The listing builds one solid part. Answer for the finished solid, in the listing's coordinates (mm). A direction names the side the tool comes from. Round coordinates to 2 decimals unless told otherwise and drop trailing zeros. Loops run counter-clockwise (first coordinate to the right, second up) from the corner with the lowest first, then second, coordinate; pieces in that order, holes last. Notation, with made-up numbers: (4, -5) -> (56, -5) arc R27 cw to (56, 30) -> close; hole circle Ø2 at (-11, 17.5). An arc over 180 degrees is marked (long way). One line per question, with ' | ' between items.
from build123d import *

# Parameters (mm, degrees)
BOX_W                   = 3.1
BOX_H                   = 13
BOX_DEPTH               = 12
BOX001_W                = 3.1
BOX001_H                = 10
BOX001_DEPTH            = 5
BOX002_W                = 3.1
BOX002_H                = 10
BOX002_DEPTH            = 5
CYLINDER_R              = 2.75
CYLINDER_DEPTH          = 3.1
CYLINDER_PITCH_ANGLE    = 90
CYLINDER001_R           = 2.75
CYLINDER001_DEPTH       = 3.06
CYLINDER001_PITCH_ANGLE = 90
PAD001_DEPTH            = 41
POCKET_DEPTH            = 41


with BuildPart() as usb:
    # Box → Box (new body)
    with BuildSketch(Plane(origin=(-130.1, 4, 14), x_dir=(1, 0, 0), z_dir=(0, 0, 1))):
        with Locations((1.55, 6.5)):
            Rectangle(BOX_W, BOX_H)
    extrude(amount=BOX_DEPTH)


with BuildPart() as obj1:
    # Box001 → Box001 (new body)
    with BuildSketch(Plane(origin=(-130.1, -5, 5), x_dir=(1, 0, 0), z_dir=(0, 0, 1))):
        with Locations((1.55, 5)):
            Rectangle(BOX001_W, BOX001_H)
    extrude(amount=BOX001_DEPTH)


with BuildPart() as obj2:
    # Box002 → Box002 (new body)
    with BuildSketch(Plane(origin=(-130.1, -5, 31), x_dir=(1, 0, 0), z_dir=(0, 0, 1))):
        with Locations((1.55, 5)):
            Rectangle(BOX002_W, BOX002_H)
    extrude(amount=BOX002_DEPTH)


with BuildPart() as passage:
    # Cylinder → Cylinder (new body)
    with BuildSketch(Plane.XY):
        Circle(CYLINDER_R)
    extrude(amount=CYLINDER_DEPTH)


with BuildPart() as passage_1:
    # Cylinder pitch: moved
    add(passage.part.rotate(Axis((0, 0, 0), (0, 1, 0)), CYLINDER_PITCH_ANGLE))


with BuildPart() as passage_2:
    # Cylinder placement: moved
    add(passage_1.part.moved(Location((-130.1, -10, 21))))


with BuildPart() as inter:
    # Cylinder001 → Cylinder001 (new body)
    with BuildSketch(Plane.XY):
        Circle(CYLINDER001_R)
    extrude(amount=CYLINDER001_DEPTH)


with BuildPart() as inter_1:
    # Cylinder001 pitch: moved
    add(inter.part.rotate(Axis((0, 0, 0), (0, 1, 0)), CYLINDER001_PITCH_ANGLE))


with BuildPart() as inter_2:
    # Cylinder001 placement: moved
    add(inter_1.part.moved(Location((-130.09, -34, 21))))


with BuildPart() as cut004:
    # Sketch → Pad001 (new body)
    with BuildSketch(Plane.XY):
        Polygon((-130.081082, 75.519378), (-130.081082, -75.526209), (-100.046493, -44.621067), (-100.046493, -60.2838), (-69.840584, -29.852762), (-69.840584, -45.201256), (-39.66638, -20.21052), (-39.66638, -34.900669), (10.150305, -0.184029), (-39.87487, 34.909859), (-39.87487, 19.507401), (-70.024222, 45.766594), (-70.024222, 29.628657), (-100.203184, 59.856933), (-100.203184, 44.62989), align=None)
    extrude(amount=PAD001_DEPTH)

    # Sketch001 → Pocket (cut)
    with BuildSketch(Plane.XY.offset(41)):
        with BuildLine():
            Line((-71.118897, 27.836128), (-98.21559, 54.89476))
            Line((-98.21559, 54.89476), (-98.042604, 39.408949))
            Line((-98.042604, 39.408949), (-127.035297, 69.474451))
            Line((-127.035297, 69.474451), (-127.035297, -69.407334))
            Line((-127.035297, -69.407334), (-98.142096, -39.664917))
            Line((-98.142096, -39.664917), (-97.815397, -55.06776))
            Line((-97.815397, -55.06776), (-70.664267, -27.971977))
            ThreePointArc((-70.664267, -27.971977), (-68.985652, -27.629399), (-68.009835, -29.037549))
            Line((-68.009835, -29.037549), (-67.738941, -40.844618))
            Line((-67.738941, -40.844618), (-37.683933, -16.715946))
            Line((-37.683933, -16.715946), (-37.564096, -30.955577))
            Line((-37.564096, -30.955577), (6.510068, -0.080506))
            Line((6.510068, -0.080506), (-37.808934, 30.841439))
            Line((-37.808934, 30.841439), (-37.808934, 14.972198))
            Line((-37.808934, 14.972198), (-68.032287, 41.206368))
            Line((-68.032287, 41.206368), (-68.032287, 29.115915))
            ThreePointArc((-68.032287, 29.115915), (-69.148192, 27.44521), (-71.118897, 27.836128))
        make_face()
    extrude(amount=-POCKET_DEPTH, mode=Mode.SUBTRACT)

    # Cut: cut Inter
    add(inter_2.part, mode=Mode.SUBTRACT)

    # Cut001: cut Passage
    add(passage_2.part, mode=Mode.SUBTRACT)

    # Cut002: cut obj2
    add(obj2.part, mode=Mode.SUBTRACT)

    # Cut003: cut obj1
    add(obj1.part, mode=Mode.SUBTRACT)

    # Cut004: cut Usb
    add(usb.part, mode=Mode.SUBTRACT)


solid = cut004.part
Q1. A cutting plane is placed at C-C on y = 50. Give the vertices of the cut face in (x, z), plus the area to 3 significant figures.
Numbers:
outline: (-130.08, 0) -> (-127.04, 0) -> (-127.04, 41) -> (-130.08, 41) -> close; (-108.26, 0) -> (-105.4, 0) -> (-105.4, 41) -> (-108.26, 41) -> close; (-100.2, 0) -> (-98.16, 0) -> (-98.16, 41) -> (-100.2, 41) -> close; (-93.31, 0) -> (-90.36, 0) -> (-90.36, 41) -> (-93.31, 41) -> close | area: 447 mm^2
Q2. A cutting plane is placed at D-D on z = 21. Give the number of separate pieces and of enclosed holes in the cut face, plus the area to 3 significant figures.
Numbers:
separate pieces: 3 | enclosed holes: 0 | area: 1,290 mm^2
Q3. For a pull along Z with two mould halves and no side action, classify faces 1 (the face through (-127.035, 1, 21)), 2 (the face through (-128.58, -9.879, 23.747)), 3 (the face through (-128.58, -31.273, 21.358)), 4 (the face through (-71, 28, 0)) as pulls with the +Z half, pulls with the -Z half, needs draft (parallel to the pull), parting line crosses it, or undercut.
Numbers:
face 1: needs draft | face 2: undercut | face 3: undercut | face 4: pulls with the -Z half
Q4. A cutting plane is placed at B-B on x = -57.5. Give the vertices of the cut face in (y, z).
Numbers:
outline: (-34.98, 0) -> (-32.62, 0) -> (-32.62, 41) -> (-34.98, 41) -> close; (32.06, 0) -> (34.86, 0) -> (34.86, 41) -> (32.06, 41) -> close
Q5. For faces 5 (the face through (-114.933, 59.858, 20.213)), 6 (the face through (-112.791, -54.744, 20.787)), 7 (the face through (-100.046, -52, 20)), determine the directions among +Z, -Z, +X, -X, +Y, -Y from which every point of the face is accessible in a straight line to the end or side of a thin tool.
Numbers:
face 5: +Z, -Z, +Y | face 6: +Z, -Z | face 7: +Z, -Z, -Y
Q6. A cutting plane is placed at A-A on y = -10. Give the vertices of the cut face in (x, z), plus the area to 3 significant figures.
Numbers:
outline: (-130.08, 0) -> (-127.04, 0) -> (-127.04, 18.25) -> (-130.08, 18.25) -> close; (-130.08, 23.75) -> (-127.04, 23.75) -> (-127.04, 41) -> (-130.08, 41) -> close; (-7.65, 0) -> (-3.94, 0) -> (-3.94, 41) -> (-7.65, 41) -> close | area: 260 mm^2
Q7. Find the intervals of material crossed by line 1 (Z direction, x = -129, y = -10); line 2 (X direction, y = -33, z = 39); line 3 (Y direction, x = -128, z = 21), in increasing order. Write a range as from..to.
Numbers:
line 1: 0..18.25, 23.75..41 | line 2: -130.08..-127.04, -75.7..-72.96, -69.84..-67.92, -57.97..-55.11, -39.67..-36.94 | line 3: -73.38..-36.75, -31.25..-12.75, -7.25..4, 17..73.37
Q8. Given pin 1 Ø10 at (y, z) = (-33, 12) entering from +X; pin 2 Ø4 at (y, z) = (-27.5, 23.5) entering from +X; pin 3 Ø1.5 at (x, z) = (-129, 34) entering from +Y, each flat-ended and moving along its own axis, determine where each tip first touches the part or whether it passes through.
Numbers:
pin 1: x = -29.76 | pin 2: x = -26.18 | pin 3: y = 75.18
